from build123d import *

# Parameters (mm, degrees)
SKETCH_1_W          = 250
SKETCH_1_H          = 150
EXTRUDE_2_DEPTH     = 200
SKETCH_3_W          = 230
SKETCH_3_H          = 130
CUT_EXTRUDE_1_DEPTH = 190
SKETCH_4_W          = 230
SKETCH_4_H          = 180
CUT_EXTRUDE_2_DEPTH = 190
SKETCH_5_R          = 40.5
SKETCH_5_R_2        = 1.55
CUT_EXTRUDE_3_DEPTH = 250
SKETCH_14_W         = 120
SKETCH_14_H         = 40
CUT_EXTRUDE_4_DEPTH = 20


with BuildPart() as part:
    # 草图1 → 凸台-拉伸2 (new body)
    with BuildSketch(Plane(origin=(0, 0, 0), x_dir=(1, 0, 0), z_dir=(0, 1, 0))):
        Rectangle(SKETCH_1_W, SKETCH_1_H)
    extrude(amount=EXTRUDE_2_DEPTH)

    # 草图3 → 切除-拉伸1 (cut)
    with BuildSketch(Plane(origin=(0, 200, 0), x_dir=(1, 0, 0), z_dir=(0, 1, 0))):
        Rectangle(SKETCH_3_W, SKETCH_3_H)
    extrude(amount=-CUT_EXTRUDE_1_DEPTH, mode=Mode.SUBTRACT)

    # 草图4 → 切除-拉伸2 (cut)
    with BuildSketch(Plane.XY.offset(75)):
        with Locations((0, 100)):
            Rectangle(SKETCH_4_W, SKETCH_4_H)
    extrude(amount=-CUT_EXTRUDE_2_DEPTH, mode=Mode.SUBTRACT)

    # 草图5 → 切除-拉伸3 (cut)
    with BuildSketch(Plane(origin=(125, 0, 0), x_dir=(0, 0, -1), z_dir=(1, 0, 0))):
        with Locations((0, 100)):
            Circle(SKETCH_5_R)
        with Locations((-24.375, 142.218738434)):
            Circle(SKETCH_5_R_2)
        with Locations((-48.75, 100)):
            Circle(SKETCH_5_R_2)
        with Locations((24.375, 142.218738434)):
            Circle(SKETCH_5_R_2)
        with Locations((48.75, 100)):
            Circle(SKETCH_5_R_2)
        with Locations((24.375, 57.781261566)):
            Circle(SKETCH_5_R_2)
        with Locations((-24.375, 57.781261566)):
            Circle(SKETCH_5_R_2)
    extrude(amount=-CUT_EXTRUDE_3_DEPTH, mode=Mode.SUBTRACT)

    # 草图10 → 旋转2 (revolve)
    with BuildSketch(Plane.XY.offset(45), mode=Mode.PRIVATE) as revolve_2_sk:
        Polygon((-75, 0), (-75, -20), (-85, -20), (-85, -10), (-95, 0), (-85, 0), align=None)
    revolve(revolve_2_sk.sketch.rotate(Axis((-75, 0, 45), (0, -1, 0)), 270), axis=Axis((-75, 0, 45), (0, -1, 0)))

    # 草图11 → 旋转4 (revolve)
    with BuildSketch(Plane.XY.offset(45), mode=Mode.PRIVATE) as revolve_4_sk:
        Polygon((75, 0), (55, 0), (65, -10), (65, -20), (75, -20), align=None)
    revolve(revolve_4_sk.sketch.rotate(Axis((75, 0, 45), (0, -1, 0)), 270), axis=Axis((75, 0, 45), (0, -1, 0)))

    # 草图12 → 旋转5 (revolve)
    with BuildSketch(Plane(origin=(0, 0, -45), x_dir=(-1, 0, 0), z_dir=(0, 0, -1)), mode=Mode.PRIVATE) as revolve_5_sk:
        Polygon((-75, 0), (-55, 0), (-65, -10), (-65, -20), (-75, -20), align=None)
    revolve(revolve_5_sk.sketch.rotate(Axis((75, 0, -45), (0, -1, 0)), 270), axis=Axis((75, 0, -45), (0, -1, 0)))

    # 草图13 → 旋转6 (revolve)
    with BuildSketch(Plane(origin=(0, 0, -45), x_dir=(-1, 0, 0), z_dir=(0, 0, -1)), mode=Mode.PRIVATE) as revolve_6_sk:
        Polygon((75, 0), (55, 0), (65, -10), (65, -20), (75, -20), align=None)
    revolve(revolve_6_sk.sketch.rotate(Axis((-75, 0, -45), (0, -1, 0)), 90), axis=Axis((-75, 0, -45), (0, -1, 0)))

    # 草图14 → 切除-拉伸4 (cut)
    with BuildSketch(Plane(origin=(0, 10, 0), x_dir=(1, 0, 0), z_dir=(0, 1, 0))):
        Rectangle(SKETCH_14_W, SKETCH_14_H)
    extrude(amount=-CUT_EXTRUDE_4_DEPTH, mode=Mode.SUBTRACT)


solid = part.part
Build history of the part. All positions in model axes, mm. A direction names the side the tool comes from. Round coordinates to 2 decimals unless told otherwise and drop trailing zeros. Write each loop counter-clockwise with the first axis right and the second up, starting at its lowest first coordinate (ties: lowest second). Pieces come first, ordered by that corner, then holes. Notation, with made-up numbers: M -0.75,35.5 L 21.25,35.5 A27 cw 21.25,53.5 Z; hole C -28.5,74.25 d1. An arc over 180 degrees is marked long. Answer in a Markdown table with one row per item.
1. Flat gauge pins, fed straight in: P1, Ø1.5, axis at x = -60, z = 43, coming from the -Y side; P2, Ø8, axis at x = 53.5, z = 68.5, coming from the -Y side; P3, Ø3, axis at y = 142.22, z = -24.38, coming from the +X side; P4, Ø3, axis at x = 95, z = 49, coming from the -Y side. Where does each tip first touch, or does it go through?
Geometry check:
| item | result |
|---|---|
| P1 | y = -5.62 |
| P2 | y = 0 |
| P3 | through |
| P4 | y = -1.1 |
2. Which spindle directions (+Z, -Z, +X, -X, +Y, -Y) get a long thin tool onto all of the face, cutting with end or side? Do faces 3 (the face through (-2, 190, -70)), 4 (the face through (75, -15, -55)), 5 (the face through (-75, -20, 45)), 6 (the face through (-10, 196, -75)), 7 (the face through (-1, 5, 20)). Say none if no direction does.
Geometry check:
| item | result |
|---|---|
| face 3 | +Z, -Z |
| face 4 | -Y |
| face 5 | +Z, -Z, +X, -X, -Y |
| face 6 | -Z, +X, -X, +Y, -Y |
| face 7 | +Y, -Y |
3. Saw through at D-D (z = 10). List the corners of the cut face in (x, y).
Geometry check:
| item | result |
|---|---|
| outline | M -125,0 L -60,0 L -60,10 L -115,10 L -115,60.75 L -125,60.75 Z; M -125,139.25 L -115,139.25 L -115,200 L -125,200 Z; M 60,0 L 125,0 L 125,60.75 L 115,60.75 L 115,10 L 60,10 Z; M 115,139.25 L 125,139.25 L 125,200 L 115,200 Z |
4. Saw through at B-B (y = 18.5). List the corners of the cut face in (x, z), and give its area (3 significant figures).
Geometry check:
| item | result |
|---|---|
| outline | M -125,-75 L -115,-75 L -115,75 L -125,75 Z; M 115,-75 L 125,-75 L 125,75 L 115,75 Z |
| area | 3,000 mm2 |
5. Saw through at C-C (x = -75). List the corners of the cut face in (y, z), and give its area (3 significant figures).
Geometry check:
| item | result |
|---|---|
| outline | M -20,-55 L -10,-55 L 0,-65 L 0,-75 L 10,-75 L 10,75 L 0,75 L 0,65 L -10,55 L -20,55 L -20,35 L -10,35 L 0,25 L 0,-25 L -10,-35 L -20,-35 Z; M 190,-75 L 200,-75 L 200,-65 L 190,-65 Z; M 190,65 L 200,65 L 200,75 L 190,75 Z |
| area | 2,700 mm2 |
6. Mould opens along X. For faces 1 (the face through (-75, -20, -45)), 2 (the face through (-84.915, -14.93, 43.698)) say: +X half, -X half, draft (parallel to the pull), parting line (faces both ways), or undercut.
Geometry check:
| item | result |
|---|---|
| face 1 | draft |
| face 2 | undercut |
7. Saw through at A-A (x = -5). List the corners of the cut face in (y, z).
Geometry check:
| item | result |
|---|---|
| outline | M 0,-75 L 10,-75 L 10,-20 L 0,-20 Z; M 0,20 L 10,20 L 10,75 L 0,75 Z; M 190,-75 L 200,-75 L 200,-65 L 190,-65 Z; M 190,65 L 200,65 L 200,75 L 190,75 Z |
8. Probe L1, parallel to X at y = 26, z = 30; L2, parallel to Y at x = 121.75, z = -48.75; L3, parallel to Y at x = 94.5, z = -19.5. List the from-to ranges inside material, lowest first. Write a range as [from, to].
Geometry check:
| item | result |
|---|---|
| L1 | [-125, -115], [115, 125] |
| L2 | [0, 98.45], [101.55, 200] |
| L3 | [0, 10] |
